Check sheet for the modelled part. Datum: model origin and axes. Units: mm. A direction names the side the tool comes from. Round coordinates to 2 decimals unless told otherwise and drop trailing zeros. Order: outer loops, then holes, each group sorted by start corner. A loop starts at its lowest first (then second) coordinate and runs counter-clockwise, first axis right, second up. Notation, with made-up numbers: (81, 83) -> (100, 83) arc R20 cw to (100, 96) -> close; hole circle Ø6 at (82, -14.75). An arc over 180 degrees is marked (long way). Answer as CSV lines item,"result". Start each with the question number.
from build123d import *

# Parameters (mm, degrees)
SALIENTE_EXTRUIR1_DEPTH      = 2
SALIENTE_EXTRUIR1_DEPTH_BACK = 10
CROQUIS1_R                   = 3.5


with BuildPart() as part:
    # Croquis1 → Saliente-Extruir1 (new, two sides: drawn at the far end of the back side and taken through both)
    with BuildSketch(Plane.XY.offset(-SALIENTE_EXTRUIR1_DEPTH_BACK)):
        with BuildLine():
            ThreePointArc((-5.08027052, 99.870870886), (-100, 0), (-5.08027052, -99.870870886))
            Line((-5.08027052, -99.870870886), (5.08027052, -99.870870886))
            ThreePointArc((5.08027052, -99.870870886), (72.4845744, -68.891120429), (100, 0))
            ThreePointArc((100, 0), (72.4845744, 68.891120429), (5.08027052, 99.870870886))
            Line((5.08027052, 99.870870886), (-5.08027052, 99.870870886))
        make_face()
        with BuildLine():
            ThreePointArc((-43.051560295, -77.15), (-48.051560295, -72.15), (-43.051560295, -67.15))
            Line((-43.051560295, -67.15), (41.948439705, -67.15))
            ThreePointArc((41.948439705, -67.15), (46.948439705, -72.15), (41.948439705, -77.15))
            Line((41.948439705, -77.15), (-43.051560295, -77.15))
        make_face(mode=Mode.SUBTRACT)
        with BuildLine():
            ThreePointArc((-70.980131723, -47.721428571), (-76.080131723, -42.621428571), (-70.980131723, -37.521428571))
            Line((-70.980131723, -37.521428571), (-10.980131723, -37.521428571))
            ThreePointArc((-10.980131723, -37.521428571), (-5.880131723, -42.621428571), (-10.980131723, -47.721428571))
            Line((-10.980131723, -47.721428571), (-70.980131723, -47.721428571))
        make_face(mode=Mode.SUBTRACT)
        with BuildLine():
            ThreePointArc((-71.465846009, -24.65), (-76.565846009, -19.55), (-71.465846009, -14.45))
            Line((-71.465846009, -14.45), (-11.465846009, -14.45))
            ThreePointArc((-11.465846009, -14.45), (-6.365846009, -19.55), (-11.465846009, -24.65))
            Line((-11.465846009, -24.65), (-71.465846009, -24.65))
        make_face(mode=Mode.SUBTRACT)
        with Locations((0, -86.821428571)):
            Circle(CROQUIS1_R, mode=Mode.SUBTRACT)
        with BuildLine():
            ThreePointArc((12.319868277, -47.721428571), (7.219868277, -42.621428571), (12.319868277, -37.521428571))
            Line((12.319868277, -37.521428571), (72.319868277, -37.521428571))
            ThreePointArc((72.319868277, -37.521428571), (77.419868277, -42.621428571), (72.319868277, -47.721428571))
            Line((72.319868277, -47.721428571), (12.319868277, -47.721428571))
        make_face(mode=Mode.SUBTRACT)
        with BuildLine():
            ThreePointArc((12.077011134, -24.65), (6.977011134, -19.55), (12.077011134, -14.45))
            Line((12.077011134, -14.45), (72.077011134, -14.45))
            ThreePointArc((72.077011134, -14.45), (77.177011134, -19.55), (72.077011134, -24.65))
            Line((72.077011134, -24.65), (12.077011134, -24.65))
        make_face(mode=Mode.SUBTRACT)
        with BuildLine():
            ThreePointArc((-71.708703152, -2.792857143), (-76.808703152, 2.307142857), (-71.708703152, 7.407142857))
            Line((-71.708703152, 7.407142857), (-11.708703152, 7.407142857))
            ThreePointArc((-11.708703152, 7.407142857), (-6.608703152, 2.307142857), (-11.708703152, -2.792857143))
            Line((-11.708703152, -2.792857143), (-71.708703152, -2.792857143))
        make_face(mode=Mode.SUBTRACT)
        with BuildLine():
            ThreePointArc((-71.465846009, 20.521428571), (-76.565846009, 25.621428571), (-71.465846009, 30.721428571))
            Line((-71.465846009, 30.721428571), (-11.465846009, 30.721428571))
            ThreePointArc((-11.465846009, 30.721428571), (-6.365846009, 25.621428571), (-11.465846009, 20.521428571))
            Line((-11.465846009, 20.521428571), (-71.465846009, 20.521428571))
        make_face(mode=Mode.SUBTRACT)
        with BuildLine():
            ThreePointArc((-71.465846009, 41.892857143), (-76.565846009, 46.992857143), (-71.465846009, 52.092857143))
            Line((-71.465846009, 52.092857143), (-11.465846009, 52.092857143))
            ThreePointArc((-11.465846009, 52.092857143), (-6.365846009, 46.992857143), (-11.465846009, 41.892857143))
            Line((-11.465846009, 41.892857143), (-71.465846009, 41.892857143))
        make_face(mode=Mode.SUBTRACT)
        with BuildLine():
            ThreePointArc((12.077011134, -2.307142857), (6.977011134, 2.792857143), (12.077011134, 7.892857143))
            Line((12.077011134, 7.892857143), (72.077011134, 7.892857143))
            ThreePointArc((72.077011134, 7.892857143), (77.177011134, 2.792857143), (72.077011134, -2.307142857))
            Line((72.077011134, -2.307142857), (12.077011134, -2.307142857))
        make_face(mode=Mode.SUBTRACT)
        with BuildLine():
            ThreePointArc((12.434153991, 20.521428571), (7.334153991, 25.621428571), (12.434153991, 30.721428571))
            Line((12.434153991, 30.721428571), (73.148439705, 30.721428571))
            ThreePointArc((73.148439705, 30.721428571), (78.248439705, 25.621428571), (73.148439705, 20.521428571))
            Line((73.148439705, 20.521428571), (12.434153991, 20.521428571))
        make_face(mode=Mode.SUBTRACT)
        with BuildLine():
            ThreePointArc((12.319868277, 41.892857143), (7.219868277, 46.992857143), (12.319868277, 52.092857143))
            Line((12.319868277, 52.092857143), (72.319868277, 52.092857143))
            ThreePointArc((72.319868277, 52.092857143), (77.419868277, 46.992857143), (72.319868277, 41.892857143))
            Line((72.319868277, 41.892857143), (12.319868277, 41.892857143))
        make_face(mode=Mode.SUBTRACT)
        with BuildLine():
            ThreePointArc((-42.322988866, 66.135714286), (-47.322988866, 71.135714286), (-42.322988866, 76.135714286))
            Line((-42.322988866, 76.135714286), (42.677011134, 76.135714286))
            ThreePointArc((42.677011134, 76.135714286), (47.677011134, 71.135714286), (42.677011134, 66.135714286))
            Line((42.677011134, 66.135714286), (-42.322988866, 66.135714286))
        make_face(mode=Mode.SUBTRACT)
        with Locations((0.177011134, 86.721428571)):
            Circle(CROQUIS1_R, mode=Mode.SUBTRACT)
    extrude(amount=SALIENTE_EXTRUIR1_DEPTH + SALIENTE_EXTRUIR1_DEPTH_BACK)


solid = part.part
1) Section check D-D on z = -7.5. Count the separate pieces of the cut face and the enclosed holes in it, then the cut area to 3 significant figures.
2) Access from +Z, -Z, +X, -X, +Y, -Y to the whole of each face (thin tool, end or side, straight path). Record for faces 3 (the face through (42, -2.307, -4)), 4 (the face through (-1, 1, 2)).
3) Mould release check, pull along Y, two halves, no side actions. Record for faces 1 (the face through (-1, 1, -10)), 2 (the face through (43, 20.521, -4)): released by +Y, released by -Y, zero draft, split by the parting line, or undercut.
4) Section check C-C on y = -72.15. Record the cut outline in (x, z), then the cut area to 3 significant figures.
5) Section check A-A on y = -20.5. Record the cut outline in (x, z).
6) Depth check by flat-ended pin: pin 1 Ø6 at (x, z) = (42, -2.5) entering from +Y; pin 2 Ø5 at (x, z) = (73.5, -1.5) entering from +Y; pin 3 Ø3.5 at (x, z) = (-6, -1.5) entering from +Y; pin 4 Ø5 at (y, z) = (27.5, -5.5) entering from +X. Enter the tip coordinate at first touch or a pass-through.
7) Material ranges on line 1 along Y through (x, z) = (0, -2.5); line 2 along X through (y, z) = (26.5, 1.75); line 3 along X through (y, z) = (-89.5, -2), recorded low to high.
8) Section check B-B on x = 0. Record the cut outline in (y, z), then the cut area to 3 significant figures.
Solutions:
1,separate pieces,"1"
1,enclosed holes,"14"
1,area,"22,500 mm^2"
2,face 3,"+Z, -Z"
2,face 4,"+Z, +X, -X, +Y, -Y"
3,face 1,"zero draft"
3,face 2,"undercut"
4,outline,"(-69.24, -10) -> (-48.05, -10) -> (-48.05, 2) -> (-69.24, 2) -> close; (46.95, -10) -> (69.24, -10) -> (69.24, 2) -> (46.95, 2) -> close"
4,area,"522 mm^2"
5,outline,"(-97.88, -10) -> (-76.48, -10) -> (-76.48, 2) -> (-97.88, 2) -> close; (-6.46, -10) -> (7.07, -10) -> (7.07, 2) -> (-6.46, 2) -> close; (77.09, -10) -> (97.88, -10) -> (97.88, 2) -> (77.09, 2) -> close"
6,pin 1,"stops at y = 92.08"
6,pin 2,"stops at y = 70.42"
6,pin 3,"stops at y = 99.87"
6,pin 4,"stops at x = 96.82"
7,line 1,"y = -99.87 to -90.32, -83.32 to -77.15, -67.15 to 66.14, 76.14 to 83.23, 90.22 to 99.87"
7,line 2,"x = -96.42 to -76.49, -6.44 to 7.41, 78.17 to 96.42"
7,line 3,"x = -44.61 to -2.25, 2.25 to 44.61"
8,outline,"(-99.87, -10) -> (-90.32, -10) -> (-90.32, 2) -> (-99.87, 2) -> close; (-83.32, -10) -> (-77.15, -10) -> (-77.15, 2) -> (-83.32, 2) -> close; (-67.15, -10) -> (66.14, -10) -> (66.14, 2) -> (-67.15, 2) -> close; (76.14, -10) -> (83.23, -10) -> (83.23, 2) -> (76.14, 2) -> close; (90.22, -10) -> (99.87, -10) -> (99.87, 2) -> (90.22, 2) -> close"
8,area,"1,990 mm^2"
